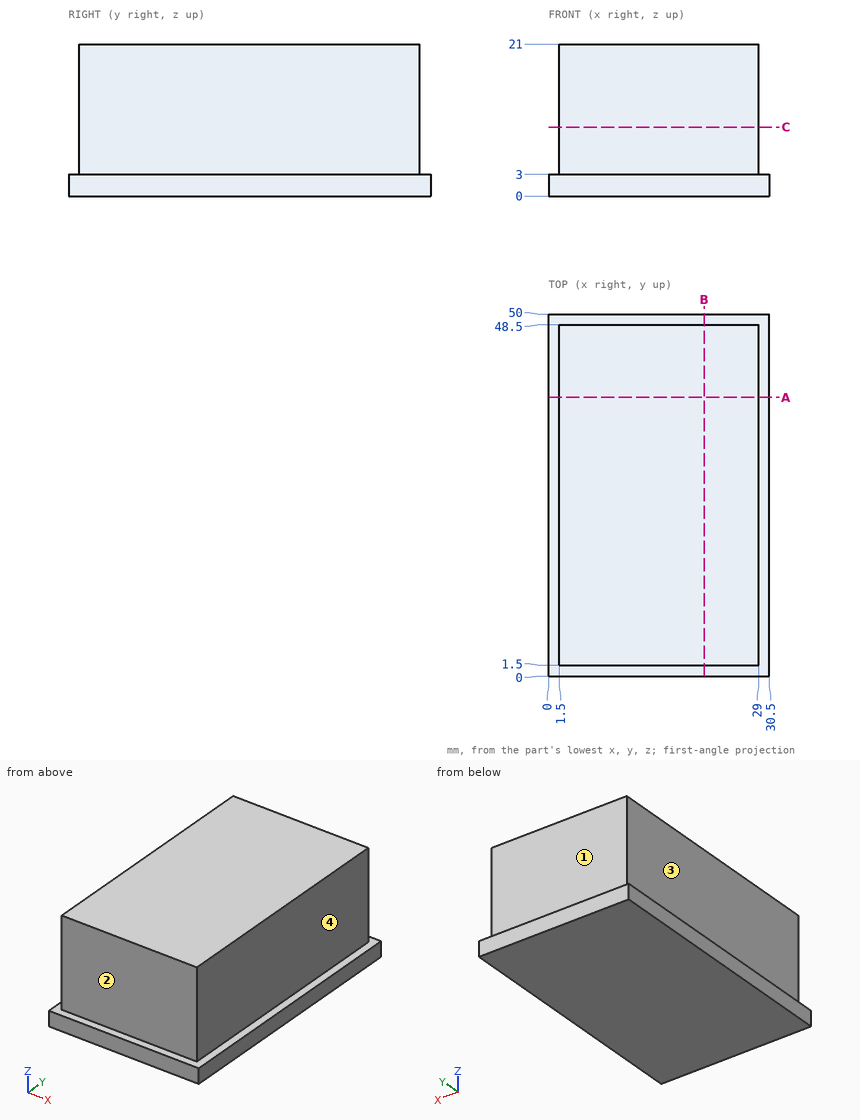
Geometry: see drawing. Coordinates: mm, zero at the bounding-box minimum. A direction names the side the tool comes from. Give positions to 0.01 mm unless a question says otherwise; leave off trailing zeros. Loops run counter-clockwise (first coordinate to the right, second up) from the corner with the lowest first, then second, coordinate; pieces in that order, holes last. Notation, with made-up numbers: (62, 14) -> (99, 14) arc R11 ccw to (99, 29) -> close; hole circle Ø11 at (77, 77.25). An arc over 180 degrees is marked (long way). Use CSV: the item, a comma, the result in double quotes.
(1) Access query for the marked faces 1, 2, 3 and 4. Directions: +Z, -Z, +X, -X, +Y, -Y. A direction counts if a zero-diameter tool reaches every point of the face in a straight line with its end or side. Return the directions, or none.
From the geometry:
face 1,"+Z, +X, -X, +Y"
face 2,"+Z, +X, -X, -Y"
face 3,"+Z, -X, +Y, -Y"
face 4,"+Z, +X, +Y, -Y"
(2) Ray query, line 1 along Y through (x, z) = (10.5, 16.5); line 2 along X through (y, z) = (31.5, 11.75). Return the intervals inside material, ascending. Write a range as [from, to].
From the geometry:
line 1,"[1.5, 48.5]"
line 2,"[1.5, 29]"
(3) Cut plane A-A (y = 38.5). Output: boundary loops of the cut face in (x, z).
From the geometry:
outline,"(0, 0) -> (30.5, 0) -> (30.5, 3) -> (29, 3) -> (29, 21) -> (1.5, 21) -> (1.5, 3) -> (0, 3) -> close"
(4) First-contact query: P1, Ø3, axis at x = 19, z = 6, coming from the -Y side; P2, Ø9, axis at y = 19, z = 14.5, coming from the +X side; P3, Ø5, axis at y = 30, z = 14, coming from the -X side; P4, Ø5, axis at x = 16.5, y = 9, coming from the -Z side. Flat tips, straight axial feed; report the tip coordinate or a pass-through.
From the geometry:
P1,"y = 1.5"
P2,"x = 29"
P3,"x = 1.5"
P4,"z = 0"
(5) Cut plane C-C (z = 9.5). Output: boundary loops of the cut face in (x, y), plus the area to 3 significant figures.
From the geometry:
outline,"(1.5, 1.5) -> (29, 1.5) -> (29, 48.5) -> (1.5, 48.5) -> close"
area,"1,290 mm^2"
(6) Cut plane B-B (x = 21.5). Output: boundary loops of the cut face in (y, z), plus the area to 3 significant figures.
From the geometry:
outline,"(0, 0) -> (50, 0) -> (50, 3) -> (48.5, 3) -> (48.5, 21) -> (1.5, 21) -> (1.5, 3) -> (0, 3) -> close"
area,"996 mm^2"
